Geometry check sheet. Reference: the model listing, model coordinates, mm. A direction names the side the tool comes from. Coordinates: 2 decimals unless noted, no trailing zeros. Order: outer loops, then holes, each group sorted by start corner. A loop starts at its lowest first (then second) coordinate and runs counter-clockwise, first axis right, second up. Notation, with made-up numbers: (48, 48.5) - (75, 48.5) arc R19 ccw to (75, 57.5) - close; hole circle Ø2 at (50.5, 6). An arc over 180 degrees is marked (long way). One line per item, written item: value. Start each with the question number.
```python
from build123d import *

# Parameters (mm, degrees)
BOSS_EXTRUDE1_DEPTH               = 3.999999999999827
BOSS_EXTRUDE2_DEPTH               = 168.00000000000006
BOSS_EXTRUDE3_DEPTH               = 33.999999999999844
BOSS_EXTRUDE4_DEPTH               = 160.00000000000026
BOSS_EXTRUDE5_DEPTH               = 33.99999999999976
BOSS_EXTRUDE6_DEPTH               = 160
CUT_EXTRUDE1_DEPTH                = 323.7305344129504
BOSS_EXTRUDE7_DEPTH               = 10
BOSS_EXTRUDE8_DEPTH               = 110.99999999999987
CUT_EXTRUDE2_DEPTH                = 320.2945688597946
CUT_EXTRUDE3_DEPTH                = 370.10495441994317
SKETCH12_R                        = 3.0000000000309623
SKETCH12_R_2                      = 2.500000000030963
SKETCH12_R_3                      = 2.192092842094092
SKETCH12_R_4                      = 2.500000000030976
CUT_EXTRUDE4_DEPTH                = 266.75584548482374
CUT_EXTRUDE11_DEPTH               = 298.4595256658518
TAP_DRILL_FOR_M33_HELICOIL1_D     = 35
TAP_DRILL_FOR_M33_HELICOIL1_DEPTH = 25
TAP_DRILL_FOR_M33_HELICOIL1_TIP   = 10.515060832982305
F_8_0_8_DIAMETER_HOLE1_D          = 8
FILLET1_START                     = -82
FILLET1_DEPTH                     = 164
FILLET1_START_2                   = -52
FILLET1_2_DEPTH                   = 104
FILLET1_3_DEPTH                   = 164
FILLET2_R                         = 6.000000000000003
FILLET3_R                         = 8.000000000000018
FILLET4_R                         = 10.000000000000002


with BuildPart() as part:
    # Sketch1 → Boss-Extrude1 (new body)
    with BuildSketch(Plane(origin=(73.22398349105087, -52.32827382689312, 1.9235e-13), x_dir=(0.581425264743257, 0.813599816567232, 0), z_dir=(0.813599816567232, -0.581425264743257, 2.1335369341433303e-15))):
        Polygon((-81.99999999999993, -57.00000000000027), (-67.00000000000007, -72.00000000000006), (67.00000000000001, -72.00000000000007), (82.00000000000031, -57.00000000000008), (82.00000000000031, 3.99999999999992), (-81.99999999999994, 3.999999999999898), align=None)
    extrude(amount=-BOSS_EXTRUDE1_DEPTH)

    # Sketch2 → Boss-Extrude2 (add)
    with BuildSketch(Plane(origin=(69.96958422478208, -50.002572767920185, 1.8081e-13), x_dir=(1.3e-16, -9e-17, 1), z_dir=(-0.8135998165672335, 0.581425264743255, 0))):
        Polygon((4.000000000000034, 82.00000000000027), (3.9999999999999107, -82.0000000000003), (-3.307e-14, -82.00000000000033), (3.0771e-13, 81.99999999999974), align=None)
    extrude(amount=BOSS_EXTRUDE2_DEPTH)

    # Sketch3 → Boss-Extrude3 (add)
    with BuildSketch(Plane(origin=(47.67687170894727, 66.71518495851329, 4e-17), x_dir=(-0.8135998165672319, 0.5814252647432572, 0), z_dir=(0.5814252647432572, 0.8135998165672319, 1.1186917952113738e-15))):
        Polygon((81.99999999999982, 1.8349e-13), (-81.9999999999999, 3.1461e-13), (-81.99999999999989, 4.000000000000039), (81.99999999999977, 3.99999999999991), align=None)
    extrude(amount=BOSS_EXTRUDE3_DEPTH)

    # Sketch4 → Boss-Extrude4 (add)
    with BuildSketch(Plane(origin=(0, 0, 0), x_dir=(-1, 0, -1.08e-15), z_dir=(1.08e-15, 1.78e-15, -1))):
        Polygon((-116.71775772643305, 22.292712515834978), (-134.16051566873062, 46.700707012851765), (-0.7301457517048301, 142.0544504307457), (16.712612190592758, 117.64645593372894), align=None)
    extrude(amount=BOSS_EXTRUDE4_DEPTH)

    # Sketch5 → Boss-Extrude5 (add)
    with BuildSketch(Plane(origin=(-47.67687170894706, -66.71518495851302, -3.148e-14), x_dir=(0.8135998165672321, -0.581425264743257, 0), z_dir=(-0.581425264743257, -0.8135998165672321, 0))):
        Polygon((-81.99999999999984, -4.049e-14), (-81.99999999999986, 3.9999999999999343), (82.00000000000009, 3.999999999999887), (82.00000000000007, -1.4474e-13), align=None)
    extrude(amount=BOSS_EXTRUDE5_DEPTH)

    # Sketch6 → Boss-Extrude6 (add)
    with BuildSketch(Plane(origin=(0, 0, 0), x_dir=(-1, 0, -1.08e-15), z_dir=(1.08e-15, 1.78e-15, -1))):
        Polygon((116.71775772643291, -22.292712515834953), (134.1605156687307, -46.70070701285208), (0.7301457517046283, -142.05445043074596), (-16.712612190593134, -117.64645593372893), align=None)
    extrude(amount=BOSS_EXTRUDE6_DEPTH)

    # Sketch7 → Cut-Extrude1 (cut, through all)
    with BuildSketch(Plane(origin=(69.96958422478208, -50.002572767920185, 1.8081e-13), x_dir=(1.3e-16, -9e-17, 1), z_dir=(-0.8135998165672335, 0.581425264743255, 0))):
        Polygon((-72.00000000000006, 55.999999999999545), (-72.00000000000001, -56.00000000000032), (-66, -56.0000000000003), (-66.0000000000001, 55.99999999999955), align=None)
    extrude(amount=-CUT_EXTRUDE1_DEPTH, mode=Mode.SUBTRACT)

    # Sketch8 → Boss-Extrude7 (add)
    with BuildSketch(Plane(origin=(-4.175e-14, -4.053e-14, -65.99999999999984), x_dir=(-1, 0, 6e-16), z_dir=(-6e-16, -5.6e-16, -1))):
        Polygon((-42.98986972440265, -94.63546428838991), (-103.45809725770025, -10.021083365397134), (-100.20369799143137, -7.695382306424205), (-39.73547045813379, -92.30976322941699), align=None)
    extrude(amount=BOSS_EXTRUDE7_DEPTH)

    # Sketch9 → Boss-Extrude8 (add)
    with BuildSketch(Plane(origin=(73.22398349105089, -52.328273826893124, 1.8922e-13), x_dir=(-1.3e-16, 9e-17, -1), z_dir=(0.8135998165672335, -0.581425264743255, 0))):
        Polygon((75.99999999999976, 51.99999999999975), (75.99999999999973, -52.00000000000022), (71.99999999999974, -52.00000000000025), (71.99999999999974, 51.99999999999975), align=None)
    extrude(amount=BOSS_EXTRUDE8_DEPTH)

    # Sketch10 → Cut-Extrude2 (cut, through all)
    with BuildSketch(Plane(origin=(66.7151849585131, -47.676871708947125, 0), x_dir=(-1.3e-15, 9.3e-16, -1), z_dir=(0.813599816567232, -0.581425264743257, -1.5973110435533651e-15))):
        Polygon((-4.000000000000134, -115.99999999999963), (155.9999999999999, -115.99999999999989), (155.9999999999999, -89.99999999999983), (-4.0000000000001315, -90.00000000000009), align=None)
    extrude(amount=-CUT_EXTRUDE2_DEPTH, mode=Mode.SUBTRACT)

    # Sketch11 → Cut-Extrude3 (cut, through all)
    with BuildSketch(Plane(origin=(-66.71518495851308, 47.67687170894687, -3.556e-14), x_dir=(5.88e-15, -4.2e-15, 1), z_dir=(-0.8135998165672317, 0.5814252647432574, 7.22907031221184e-15))):
        Polygon((-156.00000000000057, 116.00000000000004), (-156.0000000000006, 90.00000000000027), (3.9999999999994076, 89.99999999999994), (3.999999999999411, 116.00000000000033), align=None)
    extrude(amount=-CUT_EXTRUDE3_DEPTH, mode=Mode.SUBTRACT)

    # Sketch12 → Cut-Extrude4 (cut, through all)
    with BuildSketch(Plane.XY.offset(-71.99999999999953)):
        with Locations((112.5661613861435, -74.99039654371168)):
            Circle(SKETCH12_R)
        with Locations((79.7674056670706, -80.77370211065036)):
            Circle(SKETCH12_R_2)
        with Locations((118.34946695308224, -107.78915226278458)):
            Circle(SKETCH12_R_3)
        with Locations((145.3649171052164, -69.20709097677297)):
            Circle(SKETCH12_R_2)
        with Locations((106.78285581920481, -42.19164082463879)):
            Circle(SKETCH12_R_4)
    extrude(amount=-CUT_EXTRUDE4_DEPTH, mode=Mode.SUBTRACT)

    # Sketch19 → Cut-Extrude11 (cut, through all)
    with BuildSketch(Plane.XY.offset(-155.99999999999974)):
        with BuildLine():
            Line((-12.348762194736109, -115.31482156365595), (-20.484760360408547, -109.50056891622312))
            ThreePointArc((-20.484760360408547, -109.50056891622312), (-26.064860685650135, -110.42926712351874), (-25.136162478354784, -116.00936744876103))
            Line((-25.136162478354784, -116.00936744876103), (-17.00016431268235, -121.82362009619386))
            ThreePointArc((-17.00016431268235, -121.82362009619386), (-11.420063987440384, -120.89492188889805), (-12.348762194736109, -115.31482156365595))
        make_face()
        with BuildLine():
            Line((-105.09914128340088, -49.032341382924876), (-96.96314311772822, -54.84659403035742))
            ThreePointArc((-96.96314311772822, -54.84659403035742), (-96.03444491043223, -60.42669435559925), (-101.61454523567414, -61.355392562895375))
            Line((-101.61454523567414, -61.355392562895375), (-109.75054340134677, -55.54113991546282))
            ThreePointArc((-109.75054340134677, -55.54113991546282), (-110.6792416086428, -49.961039590220906), (-105.09914128340088, -49.032341382924876))
        make_face()
        with BuildLine():
            Line((101.61454523567473, 61.35539256289546), (109.75054340134734, 55.54113991546285))
            ThreePointArc((109.75054340134734, 55.54113991546285), (110.67924160864335, 49.961039590220956), (105.09914128340134, 49.0323413829248))
            Line((105.09914128340134, 49.0323413829248), (96.96314311772869, 54.84659403035741))
            ThreePointArc((96.96314311772869, 54.84659403035741), (96.0344449104327, 60.42669435559949), (101.61454523567473, 61.35539256289546))
        make_face()
        with BuildLine():
            Line((25.136162478355374, 116.00936744876108), (17.000164312682962, 121.82362009619392))
            ThreePointArc((17.000164312682962, 121.82362009619392), (11.420063987440981, 120.89492188889814), (12.348762194736782, 115.31482156365615))
            Line((12.348762194736782, 115.31482156365615), (20.484760360409194, 109.50056891622333))
            ThreePointArc((20.484760360409194, 109.50056891622333), (26.064860685651034, 110.4292671235191), (25.136162478355374, 116.00936744876108))
        make_face()
    extrude(amount=-CUT_EXTRUDE11_DEPTH, mode=Mode.SUBTRACT)

    # Tap Drill for M33 Helicoil1
    with Locations(Plane(origin=(0, 0, 0), x_dir=(-1, 0, -1.08e-15), z_dir=(1.08e-15, 1.78e-15, -1))):
        with Locations((0, 0)):
            Hole(TAP_DRILL_FOR_M33_HELICOIL1_D / 2, depth=TAP_DRILL_FOR_M33_HELICOIL1_DEPTH)
            with Locations((0, 0, -(TAP_DRILL_FOR_M33_HELICOIL1_DEPTH + TAP_DRILL_FOR_M33_HELICOIL1_TIP / 2))):  # 118° drill point
                Cone(0, TAP_DRILL_FOR_M33_HELICOIL1_D / 2, TAP_DRILL_FOR_M33_HELICOIL1_TIP, mode=Mode.SUBTRACT)

    # 8.0 _8_ Diameter Hole1 (through all)
    with Locations(Plane(origin=(0, 0, 0), x_dir=(-1, 0, -1.08e-15), z_dir=(1.08e-15, 1.78e-15, -1))):
        with Locations((10.507020801, 63.131628475), (63.131628475, -10.507020801), (-63.131628475, 10.507020801), (-10.507020801, -63.131628475)):
            Hole(F_8_0_8_DIAMETER_HOLE1_D / 2)

    # Fillet1: read off the stored shape, not the designer's step
    # Fillet1 outline → Fillet1 (add)
    with BuildSketch(Plane(origin=(0, 0, 0), x_dir=(0.5814252647432568, 0.813599816567232, 0), z_dir=(0.813599816567232, -0.581425264743257, 0)).offset(FILLET1_START)):
        with BuildLine():
            Line((-90, -156), (-90, -152))
            ThreePointArc((-90, -152), (-91.171572875, -154.828427125), (-94, -156))
            Line((-94, -156), (-90, -156))
        make_face()
        with BuildLine():
            ThreePointArc((-86, -4), (-84.828427125, -1.171572875), (-82, 0))
            Line((-82, 0), (-86, 0))
            Line((-86, 0), (-86, -4))
        make_face()
        with BuildLine():
            ThreePointArc((82, 0), (84.828427125, -1.171572875), (86, -4))
            Line((86, -4), (86, 0))
            Line((86, 0), (82, 0))
        make_face()
        with BuildLine():
            ThreePointArc((94, -156), (91.171572875, -154.828427125), (90, -152))
            Line((90, -152), (90, -156))
            Line((90, -156), (94, -156))
        make_face()
    extrude(amount=FILLET1_DEPTH)

    # Fillet1 2 outline → Fillet1 2 (add)
    with BuildSketch(Plane(origin=(0, 0, 0), x_dir=(0.813599816567232, -0.581425264743257, 0), z_dir=(0.581425264743257, 0.813599816567232, 0)).offset(FILLET1_START_2)):
        with BuildLine():
            Line((90, 72), (90, 68))
            ThreePointArc((90, 68), (91.171572875, 70.828427125), (94, 72))
            Line((94, 72), (90, 72))
        make_face()
        with BuildLine():
            ThreePointArc((86, 4), (84.828427125, 1.171572875), (82, 0))
            Line((82, 0), (86, 0))
            Line((86, 0), (86, 4))
        make_face()
    extrude(amount=FILLET1_2_DEPTH)

    # Fillet1 3 outline → Fillet1 3 (add)
    with BuildSketch(Plane(origin=(0, 0, 0), x_dir=(0.813599816567232, -0.581425264743257, 0), z_dir=(0.581425264743257, 0.813599816567232, 0)).offset(FILLET1_START)):
        with BuildLine():
            ThreePointArc((86, 4), (84.828427125, 1.171572875), (82, 0))
            Line((82, 0), (86, 0))
            Line((86, 0), (86, 4))
        make_face()
    extrude(amount=FILLET1_3_DEPTH)

    # Fillet2
    fillet2_edges = [part.edges().sort_by_distance(p)[0] for p in [
        (193.7676768966628, -74.55928775189841, -73.99999999999957),
        (133.2994493633643, -159.17366867489068, -73.99999999999957),
    ]]
    fillet(fillet2_edges, radius=FILLET2_R)

    # Fillet3
    fillet3_edges = [part.edges().sort_by_distance(p)[0] for p in [
        (69.96958422478254, -50.00257276792064, -75.99999999999986),
        (-52.32827382689307, -73.223983491051, 4.000000000000262),
        (52.32827382689298, 73.22398349105063, 3.999999999998779),
        (50.00257276792032, 69.96958422478224, -160.00000000000009),
        (73.22398349105097, -52.32827382689296, 4.000000000000101),
        (-50.002572767919716, -69.96958422478166, -160.00000000000017),
    ]]
    fillet(fillet3_edges, radius=FILLET3_R)

    # Fillet4
    fillet4_edges = [part.edges().sort_by_distance(p)[0] for p in [
        (-134.16051566873054, -46.700707012851794, -157.99999999999994),
        (134.1605156687308, 46.70070701285205, -158.0000000000009),
        (0.7301457517050038, 142.054450430746, -158.00000000000028),
        (-0.7301457517044567, -142.05445043074567, -158.00000000000006),
    ]]
    fillet(fillet4_edges, radius=FILLET4_R)


solid = part.part
```
Q1. Release check for a two-part mould opening along X. For faces 1 (the flat face through (60, 86, -156)), 2 (the cylindrical face through (70.7, -51.94, 1.59)), 3 (the cylindrical face through (68.37, -50.27, -1.2)) record: released by +X, released by -X, zero draft, split by the parting line, or undercut.
Q2. Cross-section at C-C, the plane x = 162. Enter the section's corners in (y, z).
Q3. Material ranges on probe 1 along Z at (x, y) = (-30.5, -15); probe 2 along X at (y, z) = (-89, -54.5); probe 3 along Y at (x, z) = (79.5, -40.5), recorded low to high.
Q4. Set-up check for faces 4 (the flat face through (120, -85, -76)), 5 (the flat face through (12, 15, 0)), 6 (the cylindrical face through (52.263, 71.158, -157.594)), 7 (the flat face through (36, -101, -72)): record each of +Z, -Z, +X, -X, +Y, -Y from which the full face is reachable in a straight line by a thin tool's end or side.
Q5. Gauge pin test, flat ends, axial feed: P1, Ø3, axis at x = 106.5, y = -3.5, coming from the -Z side; P2, Ø4.5, axis at x = 145.36, y = -69.21, coming from the +Z side; P3, Ø10, axis at x = 77, z = -142.5, coming from the +Y side; P4, Ø12, axis at x = -67.5, z = -106, coming from the -Y side. Record the tip position at first contact, or that the pin passes through.
Q6. Cross-section at A-A, the plane z = -143. Enter the section's corners in (x, y), and give its area (3 significant figures).
Q7. Cross-section at B-B, the plane z = -14.5. Enter the section's corners in (x, y), and give its area (3 significant figures).
Check result:
1. face 1: zero draft
1. face 2: released by +X
1. face 3: undercut
2. outline: (-119.01, -76) - (-51.86, -76) - (-51.86, -72) - (-119.01, -72) - close
3. probe 1: z = 0 to 4
3. probe 2: x = -30.25 to -23.37, 42.1 to 47.02
3. probe 3: y = -43.55 to -36.67, 48.89 to 53.81
4. face 4: -Z, +X, -Y
4. face 5: -Z
4. face 6: -Z, -X
4. face 7: -Z, -Y
5. P1: stops at z = -72
5. P2: passes through
5. P3: stops at y = 59.17
5. P4: stops at y = -66.67
6. outline: (-119.04, -25.55) - (14.39, -120.9) - (16.71, -117.65) - (-116.72, -22.29) - close; (-16.71, 117.65) - (116.72, 22.29) - (119.04, 25.55) - (-14.39, 120.9) - close
6. area: 1,310 mm2
7. outline: (-119.04, -25.55) - (14.39, -120.9) - (16.71, -117.65) - (-116.72, -22.29) - close; (-16.71, 117.65) - (116.72, 22.29) - (119.04, 25.55) - (-14.39, 120.9) - close; (22.29, -116.72) - (25.55, -119.04) - (120.9, 14.39) - (117.65, 16.71) - close
7. area: 1,970 mm2
